from build123d import *

# Parameters (mm, degrees)
CUT_EXTRUDE1_REACH             = 60.152
SKETCH3_R                      = 1.5
CUT_EXTRUDE2_DEPTH             = 0.79375
CUT_EXTRUDE2_DIRECTION_2_REACH = 56.45
CUT_EXTRUDE3_REACH             = 56.45
SKETCH5_R                      = 1.2


with BuildPart() as part:
    # Sketch1 → Revolve1 (revolve)
    with BuildSketch(Plane.XY, mode=Mode.PRIVATE) as revolve1_sk:
        Polygon((0, 0), (0, 55.4), (4.41, 55.4), (4.41, 6.4), (7, 6.4), (7, 3.9), (12.5, 3.9), (12.5, 0), align=None)
    revolve(revolve1_sk.sketch.rotate(Axis((0, 0, 0), (0, 1, 0)), 90), axis=Axis((0, 0, 0), (0, 1, 0)))

    # Sketch2 → Cut-Extrude1 (cut, up to next)
    with BuildSketch(Plane(origin=(0, 55.4, 0), x_dir=(1, 0, 0), z_dir=(0, 1, 0)), mode=Mode.PRIVATE) as cut_extrude1_sk1:
        with BuildLine():
            Line((-0.935, -1.435), (-0.935, -2.35))
            ThreePointArc((-0.935, -2.35), (0, -2.529174767), (0.935, -2.35))
            Line((0.935, -2.35), (0.935, -1.435))
            ThreePointArc((0.935, -1.435), (1.081446609, -1.081446609), (1.435, -0.935))
            Line((1.435, -0.935), (2.35, -0.935))
            ThreePointArc((2.35, -0.935), (2.529174767, 0), (2.35, 0.935))
            Line((2.35, 0.935), (1.435, 0.935))
            ThreePointArc((1.435, 0.935), (1.081446609, 1.081446609), (0.935, 1.435))
            Line((0.935, 1.435), (0.935, 2.35))
            ThreePointArc((0.935, 2.35), (0, 2.529174767), (-0.935, 2.35))
            Line((-0.935, 2.35), (-0.935, 1.435))
            ThreePointArc((-0.935, 1.435), (-1.081446609, 1.081446609), (-1.435, 0.935))
            Line((-1.435, 0.935), (-2.35, 0.935))
            ThreePointArc((-2.35, 0.935), (-2.529174767, 0), (-2.35, -0.935))
            Line((-2.35, -0.935), (-1.435, -0.935))
            ThreePointArc((-1.435, -0.935), (-1.081446609, -1.081446609), (-0.935, -1.435))
        make_face()
    cut_extrude1_tool1 = extrude(cut_extrude1_sk1.sketch, amount=-CUT_EXTRUDE1_REACH, mode=Mode.PRIVATE) & part.part
    # Sketch2 → Cut-Extrude1 (cut, up to next)
    with BuildSketch(Plane(origin=(0, 55.4, 0), x_dir=(1, 0, 0), z_dir=(0, 1, 0)), mode=Mode.PRIVATE) as cut_extrude1_sk2:
        with BuildLine():
            Line((1.055, 2.430041552), (1.055, 1.435))
            ThreePointArc((1.055, 1.435), (1.166299423, 1.166299423), (1.435, 1.055))
            Line((1.435, 1.055), (2.430041552, 1.055))
            ThreePointArc((2.430041552, 1.055), (2.649174767, 0), (2.430041552, -1.055))
            Line((2.430041552, -1.055), (1.435, -1.055))
            ThreePointArc((1.435, -1.055), (1.166299423, -1.166299423), (1.055, -1.435))
            Line((1.055, -1.435), (1.055, -2.430041552))
            ThreePointArc((1.055, -2.430041552), (0, -2.649174767), (-1.055, -2.430041552))
            Line((-1.055, -2.430041552), (-1.055, -1.435))
            ThreePointArc((-1.055, -1.435), (-1.166299423, -1.166299423), (-1.435, -1.055))
            Line((-1.435, -1.055), (-2.430041552, -1.055))
            ThreePointArc((-2.430041552, -1.055), (-2.649174767, 0), (-2.430041552, 1.055))
            Line((-2.430041552, 1.055), (-1.435, 1.055))
            ThreePointArc((-1.435, 1.055), (-1.166299423, 1.166299423), (-1.055, 1.435))
            Line((-1.055, 1.435), (-1.055, 2.430041552))
            ThreePointArc((-1.055, 2.430041552), (0, 2.649174767), (1.055, 2.430041552))
        make_face()
    cut_extrude1_tool2 = extrude(cut_extrude1_sk2.sketch, amount=-CUT_EXTRUDE1_REACH, mode=Mode.PRIVATE) & part.part
    add(cut_extrude1_tool1.solids().sort_by_distance((0, 55.4, 0))[0], mode=Mode.SUBTRACT)
    add(cut_extrude1_tool2.solids().sort_by_distance((0, 55.4, 0))[0], mode=Mode.SUBTRACT)

    # Sketch3 → Cut-Extrude2 (cut)
    with BuildSketch(Plane(origin=(0, 3.9, 0), x_dir=(1, 0, 0), z_dir=(0, 1, 0))):
        with Locations(Location((0, 8, 0), (0, 0, 314.048625674))):
            Circle(SKETCH3_R)
        with Locations(Location((0, -8, 0), (0, 0, 90))):
            Circle(SKETCH3_R)
        with Locations(Location((-8, 0, 0), (0, 0, 44.048625674))):
            Circle(SKETCH3_R)
        with Locations(Location((8, 0, 0), (0, 0, 90))):
            Circle(SKETCH3_R)
    extrude(amount=-CUT_EXTRUDE2_DEPTH, mode=Mode.SUBTRACT)

    # Cut-Extrude2 direction 2: up to this face of the body (flat: up to its plane)
    cut_extrude2_direction_2_end = Plane(part.part.faces().sort_by_distance((0, 6.4, 4.607989899))[0])
    # Sketch3 → Cut-Extrude2 direction 2 (cut, up to the picked face)
    with BuildSketch(Plane(origin=(0, 3.9, 0), x_dir=(1, 0, 0), z_dir=(0, 1, 0)), mode=Mode.PRIVATE) as cut_extrude2_direction_2_sk1:
        with Locations(Location((0, 8, 0), (0, 0, 314.048625674))):
            Circle(SKETCH3_R)
    cut_extrude2_direction_2_tool1 = split(extrude(cut_extrude2_direction_2_sk1.sketch, amount=CUT_EXTRUDE2_DIRECTION_2_REACH, mode=Mode.PRIVATE), bisect_by=cut_extrude2_direction_2_end, keep=Keep.BOTH, mode=Mode.PRIVATE)
    # Sketch3 → Cut-Extrude2 direction 2 (cut, up to the picked face)
    with BuildSketch(Plane(origin=(0, 3.9, 0), x_dir=(1, 0, 0), z_dir=(0, 1, 0)), mode=Mode.PRIVATE) as cut_extrude2_direction_2_sk2:
        with Locations(Location((0, -8, 0), (0, 0, 90))):
            Circle(SKETCH3_R)
    cut_extrude2_direction_2_tool2 = split(extrude(cut_extrude2_direction_2_sk2.sketch, amount=CUT_EXTRUDE2_DIRECTION_2_REACH, mode=Mode.PRIVATE), bisect_by=cut_extrude2_direction_2_end, keep=Keep.BOTH, mode=Mode.PRIVATE)
    # Sketch3 → Cut-Extrude2 direction 2 (cut, up to the picked face)
    with BuildSketch(Plane(origin=(0, 3.9, 0), x_dir=(1, 0, 0), z_dir=(0, 1, 0)), mode=Mode.PRIVATE) as cut_extrude2_direction_2_sk3:
        with Locations(Location((-8, 0, 0), (0, 0, 44.048625674))):
            Circle(SKETCH3_R)
    cut_extrude2_direction_2_tool3 = split(extrude(cut_extrude2_direction_2_sk3.sketch, amount=CUT_EXTRUDE2_DIRECTION_2_REACH, mode=Mode.PRIVATE), bisect_by=cut_extrude2_direction_2_end, keep=Keep.BOTH, mode=Mode.PRIVATE)
    # Sketch3 → Cut-Extrude2 direction 2 (cut, up to the picked face)
    with BuildSketch(Plane(origin=(0, 3.9, 0), x_dir=(1, 0, 0), z_dir=(0, 1, 0)), mode=Mode.PRIVATE) as cut_extrude2_direction_2_sk4:
        with Locations(Location((8, 0, 0), (0, 0, 90))):
            Circle(SKETCH3_R)
    cut_extrude2_direction_2_tool4 = split(extrude(cut_extrude2_direction_2_sk4.sketch, amount=CUT_EXTRUDE2_DIRECTION_2_REACH, mode=Mode.PRIVATE), bisect_by=cut_extrude2_direction_2_end, keep=Keep.BOTH, mode=Mode.PRIVATE)
    add(cut_extrude2_direction_2_tool1.solids().sort_by(Axis((0, 3.9, -8), (0, 1, 0)))[0], mode=Mode.SUBTRACT)
    add(cut_extrude2_direction_2_tool2.solids().sort_by(Axis((0, 3.9, 8), (0, 1, 0)))[0], mode=Mode.SUBTRACT)
    add(cut_extrude2_direction_2_tool3.solids().sort_by(Axis((-8, 3.9, 0), (0, 1, 0)))[0], mode=Mode.SUBTRACT)
    add(cut_extrude2_direction_2_tool4.solids().sort_by(Axis((8, 3.9, 0), (0, 1, 0)))[0], mode=Mode.SUBTRACT)

    # Sketch5 → Cut-Extrude3 (cut, up to next)
    with BuildSketch(Plane(origin=(0, 3.9, 0), x_dir=(1, 0, 0), z_dir=(0, 1, 0)), mode=Mode.PRIVATE) as cut_extrude3_sk1:
        with Locations(Location((8, 0, 0), (0, 0, 90))):
            Circle(SKETCH5_R)
    cut_extrude3_tool1 = extrude(cut_extrude3_sk1.sketch, amount=-CUT_EXTRUDE3_REACH, mode=Mode.PRIVATE) & part.part
    # Sketch5 → Cut-Extrude3 (cut, up to next)
    with BuildSketch(Plane(origin=(0, 3.9, 0), x_dir=(1, 0, 0), z_dir=(0, 1, 0)), mode=Mode.PRIVATE) as cut_extrude3_sk2:
        with Locations(Location((0, 8, 0), (0, 0, 270))):
            Circle(SKETCH5_R)
    cut_extrude3_tool2 = extrude(cut_extrude3_sk2.sketch, amount=-CUT_EXTRUDE3_REACH, mode=Mode.PRIVATE) & part.part
    # Sketch5 → Cut-Extrude3 (cut, up to next)
    with BuildSketch(Plane(origin=(0, 3.9, 0), x_dir=(1, 0, 0), z_dir=(0, 1, 0)), mode=Mode.PRIVATE) as cut_extrude3_sk3:
        with Locations(Location((-8, 0, 0), (0, 0, 270))):
            Circle(SKETCH5_R)
    cut_extrude3_tool3 = extrude(cut_extrude3_sk3.sketch, amount=-CUT_EXTRUDE3_REACH, mode=Mode.PRIVATE) & part.part
    # Sketch5 → Cut-Extrude3 (cut, up to next)
    with BuildSketch(Plane(origin=(0, 3.9, 0), x_dir=(1, 0, 0), z_dir=(0, 1, 0)), mode=Mode.PRIVATE) as cut_extrude3_sk4:
        with Locations(Location((0, -8, 0), (0, 0, 90))):
            Circle(SKETCH5_R)
    cut_extrude3_tool4 = extrude(cut_extrude3_sk4.sketch, amount=-CUT_EXTRUDE3_REACH, mode=Mode.PRIVATE) & part.part
    add(cut_extrude3_tool1.solids().sort_by_distance((8, 3.9, 0))[0], mode=Mode.SUBTRACT)
    add(cut_extrude3_tool2.solids().sort_by_distance((0, 3.9, -8))[0], mode=Mode.SUBTRACT)
    add(cut_extrude3_tool3.solids().sort_by_distance((-8, 3.9, 0))[0], mode=Mode.SUBTRACT)
    add(cut_extrude3_tool4.solids().sort_by_distance((0, 3.9, 8))[0], mode=Mode.SUBTRACT)


solid = part.part
The listing builds one solid part. Answer for the finished solid, in the listing's coordinates (mm). A direction names the side the tool comes from. Round coordinates to 2 decimals unless told otherwise and drop trailing zeros. Order: outer loops, then holes, each group sorted by start corner. A loop starts at its lowest first (then second) coordinate and runs counter-clockwise, first axis right, second up. Notation, with made-up numbers: M 42,80 L 86,80 A21 ccw 86,108 Z; hole C -1,-3.75 d3. An arc over 180 degrees is marked long. Answer in a Markdown table with one row per item. Add a question column.
1) The part is cut by section D-D on x = -3.75. Determine the outline of the cut face in (y, z).
2) The part is cut by section A-A on y = 36. Determine the outline of the cut face in (x, z) (3 decimals).
3) Which of the six approach directions +Z, -Z, +X, -X, +Y, -Y give full straight-line access (tool end or side, diameter ignored) to faces 4 (the face through (-0.02, 28.09, -2.65)), 5 (the face through (0, 6.4, 5)), 6 (the face through (5, 5.1, -4.9))?
4) Flat-ended cylindrical pins translate along their axes: pin 1 Ø2.5 at (x, z) = (-0.5, -8.5) entering from +Y; pin 2 Ø6 at (x, y) = (-9, 45) entering from +Z; pin 3 Ø1.1 at (y, z) = (36, 2) entering from +X; pin 4 Ø10 at (x, y) = (3, 40) entering from +Z. Find the tip coordinate at first contact, or state that the pin passes through.
5) The part is cut by section C-C on x = -8. Determine the outline of the cut face in (y, z), plus the area to 3 significant figures.
6) Determine the mould class of faces 1 (the face through (-5, 5.1, 4.9)), 2 (the face through (5.4, 3.9, 5.4)), 3 (the face through (-2, 28, 1.055)) for opening direction X: pulls with the +X half, pulls with the -X half, needs draft (parallel to the pull), parting line crosses it, or undercut.
7) The part is cut by section B-B on z = -8. Determine the outline of the cut face in (x, y).
8) Consider line 1 along Z through (x, y) = (-0.25, 31.5); line 2 along Y through (x, z) = (-2.5, 10.75); line 3 along Z through (x, y) = (1.75, 16) (3 decimals). Determine where each line is inside the solid, lowest interval first. Write a range as from..to.
Findings below:
| question | item | result |
|---|---|---|
| 1 | outline | M 0,-11.92 L 3.9,-11.92 L 3.9,-5.91 L 6.4,-5.91 L 6.4,-2.32 L 55.4,-2.32 L 55.4,2.32 L 6.4,2.32 L 6.4,5.91 L 3.9,5.91 L 3.9,11.92 L 0,11.92 Z |
| 2 | outline | C 0,0 d8.82; hole M -2.43,-1.055 L -1.435,-1.055 A0.38 cw -1.055,-1.435 L -1.055,-2.43 A2.649 ccw 1.055,-2.43 L 1.055,-1.435 A0.38 cw 1.435,-1.055 L 2.43,-1.055 A2.649 ccw 2.43,1.055 L 1.435,1.055 A0.38 cw 1.055,1.435 L 1.055,2.43 A2.649 ccw -1.055,2.43 L -1.055,1.435 A0.38 cw -1.435,1.055 L -2.43,1.055 A2.649 ccw Z |
| 3 | face 4 | +Y, -Y |
| 3 | face 5 | +Y |
| 3 | face 6 | -Z, +X, +Y |
| 4 | pin 1 | stops at y = 3.9 |
| 4 | pin 2 | passes through |
| 4 | pin 3 | stops at x = 4.16 |
| 4 | pin 4 | stops at z = 4.41 |
| 5 | outline | M 0,-9.6 L 3.9,-9.6 L 3.9,-1.5 L 3.11,-1.5 L 3.11,-1.2 L 0,-1.2 Z; M 0,1.2 L 3.11,1.2 L 3.11,1.5 L 3.9,1.5 L 3.9,9.6 L 0,9.6 Z |
| 5 | area | 65.1 mm² |
| 6 | face 1 | pulls with the -X half |
| 6 | face 2 | needs draft |
| 6 | face 3 | undercut |
| 7 | outline | M -9.6,0 L -1.2,0 L -1.2,3.11 L -1.5,3.11 L -1.5,3.9 L -9.6,3.9 Z; M 1.2,0 L 9.6,0 L 9.6,3.9 L 1.5,3.9 L 1.5,3.11 L 1.2,3.11 Z |
| 8 | line 1 | z = -4.4..-2.64, 2.64..4.4 |
| 8 | line 2 | y = 0..3.9 |
| 8 | line 3 | z = -4.048..-1.055, 1.055..4.048 |
